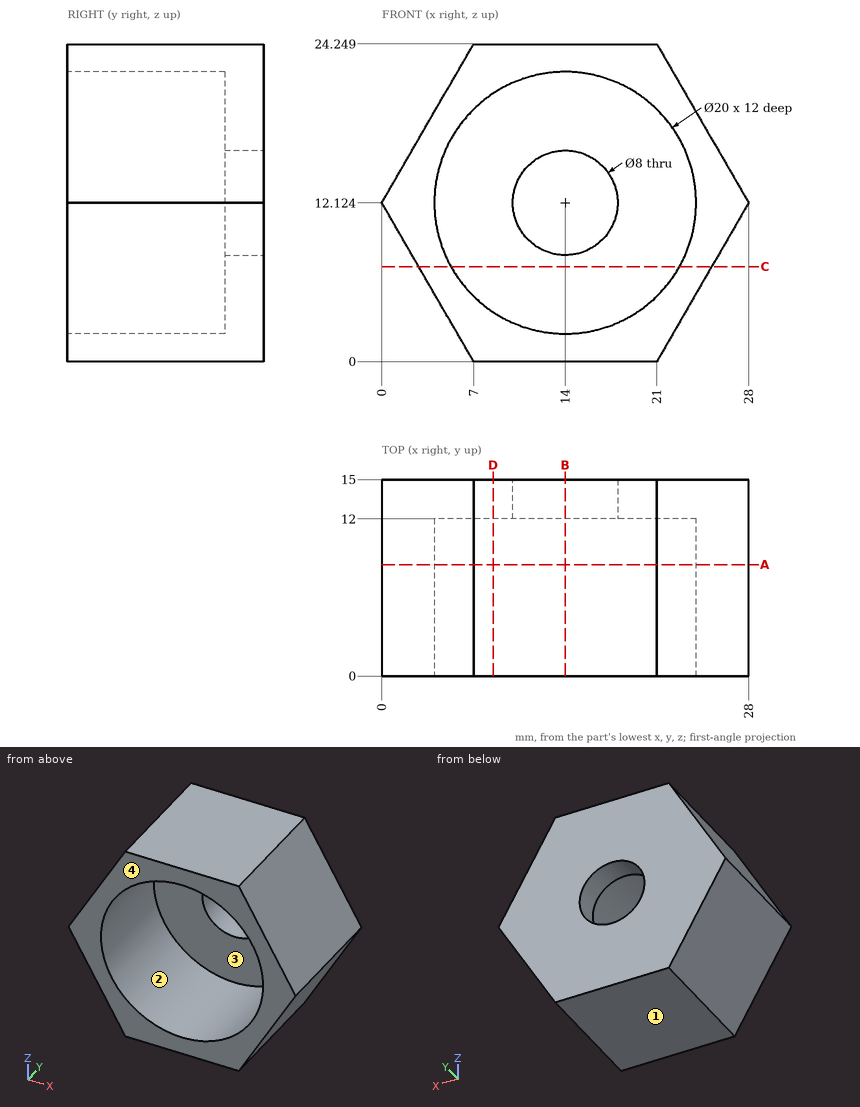
Job drawing, mm, ordinate dimensions from the low corner. One solid piece. Coordinates: 2 decimals unless noted, no trailing zeros. Order: outer loops, then holes, each group sorted by start corner. A loop starts at its lowest first (then second) coordinate and runs counter-clockwise, first axis right, second up. Notation, with made-up numbers: M -20.5,87 L 23.5,87 A17 ccw 23.5,111 Z; hole C -15,54 d10. An arc over 180 degrees is marked long. Return JSON: item names as keys, results as strings.
1. Pull direction Z, two halves, no side cores. Call the marked faces 1, 2, 3 and 4: +Z half, -Z half, draft (parallel to the pull), parting line (faces both ways), or undercut.
Ans:
{"face 1": "-Z half", "face 2": "undercut", "face 3": "undercut", "face 4": "draft"}
2. Saw through at C-C (z = 7.25). Give the cut face in (x, y).
Ans:
{"outline": "M 2.81,0 L 5.27,0 L 5.27,12 L 22.73,12 L 22.73,0 L 25.19,0 L 25.19,15 L 2.81,15 Z"}
3. Saw through at A-A (y = 8.5). Give the cut face in (x, z) (1 decimal), and give its area (3 significant figures).
Ans:
{"outline": "M 0,12.1 L 7,0 L 21,0 L 28,12.1 L 21,24.2 L 7,24.2 Z; hole C 14,12.1 d20", "area": "195 mm^2"}
4. Flat gauge pins, fed straight in: pin 1 (1 mm diameter, centred on y = 8, z = 13.5, fed in from -X) (1 decimal); pin 2 (13 mm diameter, centred on x = 14, z = 12.12, fed in from -Y); pin 3 (3 mm diameter, centred on y = 1.5, z = 8.5, fed in from -X). Where does each tip first touch, or does it go through?
Ans:
{"pin 1": "x = 0.5", "pin 2": "y = 12", "pin 3": "x = 1.23"}
5. Saw through at B-B (x = 14). Give the cut face in (y, z) (1 decimal).
Ans:
{"outline": "M 0,0 L 15,0 L 15,8.1 L 12,8.1 L 12,2.1 L 0,2.1 Z; M 0,22.1 L 12,22.1 L 12,16.1 L 15,16.1 L 15,24.2 L 0,24.2 Z"}
6. Drill centre lines: probe 1 along Z at (x, y) = (14, 12.8) (1 decimal); probe 2 along Z at (x, y) = (14, 6) (1 decimal); probe 3 along Y at (x, z) = (21.5, 10.5). Where is each one in solid material? Low to high.
Ans:
{"probe 1": "0 to 8.1, 16.1 to 24.2", "probe 2": "0 to 2.1, 22.1 to 24.2", "probe 3": "12 to 15"}
7. Saw through at D-D (x = 8.5). Give the cut face in (y, z), and give its area (3 significant figures).
Ans:
{"outline": "M 0,0 L 15,0 L 15,24.25 L 0,24.25 L 0,20.48 L 12,20.48 L 12,3.77 L 0,3.77 Z", "area": "163 mm^2"}
